from build123d import *

# Parameters (mm, degrees)
SKETCH2_W           = 40
SKETCH2_H           = 25
BOSS_EXTRUDE1_DEPTH = 15
SKETCH3_W           = 25
SKETCH3_H           = 12
CUT_EXTRUDE1_DEPTH  = 5
CUT_EXTRUDE2_DEPTH  = 4.8
SKETCH7_W           = 40
SKETCH7_H           = 25
CUT_EXTRUDE3_DEPTH  = 5


with BuildPart() as part:
    # Sketch2 → Boss-Extrude1 (new body)
    with BuildSketch(Plane.XY):
        with Locations((2.333785617, 1.285617368)):
            Rectangle(SKETCH2_W, SKETCH2_H)
    extrude(amount=BOSS_EXTRUDE1_DEPTH)

    # Sketch3 → Cut-Extrude1 (cut)
    with BuildSketch(Plane.XY.offset(15)):
        with Locations((-0.166214383, 1.285617368)):
            Rectangle(SKETCH3_W, SKETCH3_H)
    extrude(amount=-CUT_EXTRUDE1_DEPTH, mode=Mode.SUBTRACT)

    # Sketch5 → Cut-Extrude2 (cut)
    with BuildSketch(Plane.XY.offset(10)):
        with BuildLine():
            Line((10.563785617, -1.134382632), (10.563785617, 3.705617368))
            Line((10.563785617, 3.705617368), (-6.554265375, 4.705617368))
            ThreePointArc((-6.554265375, 4.705617368), (-11.666214383, 1.285617368), (-6.554265375, -2.134382632))
            Line((-6.554265375, -2.134382632), (10.563785617, -1.134382632))
        make_face()
    extrude(amount=-CUT_EXTRUDE2_DEPTH, mode=Mode.SUBTRACT)

    # Sketch7 → Cut-Extrude3 (cut)
    with BuildSketch(Plane.XY.offset(15)):
        with Locations((2.333785617, 1.285617368)):
            Rectangle(SKETCH7_W, SKETCH7_H)
    extrude(amount=-CUT_EXTRUDE3_DEPTH, mode=Mode.SUBTRACT)


solid = part.part
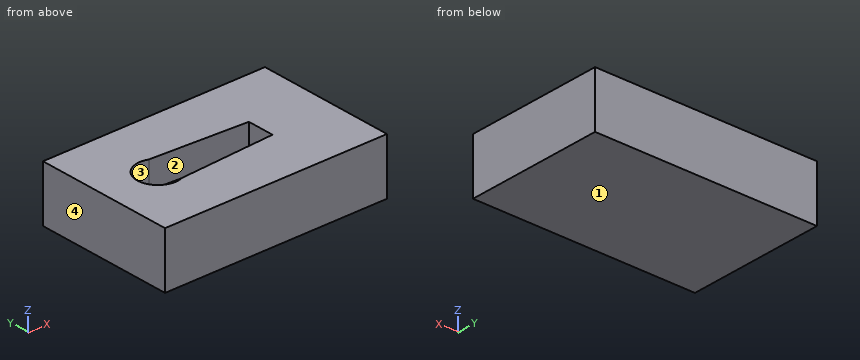
Source: CAD feature listing. Evaluate the final solid. Frame: model axes, mm. Face numbers are marked on the shaded views. Round coordinates to 2 decimals unless told otherwise and drop trailing zeros. Order: outer loops, then holes, each group sorted by start corner. A loop starts at its lowest first (then second) coordinate and runs counter-clockwise, first axis right, second up. Notation, with made-up numbers: (-7, 36) -> (38, 36) arc R13 ccw to (38, 42) -> close; hole circle Ø7 at (-4, 39). An arc over 180 degrees is marked (long way). Answer as CSV lines item,"result".
Item 1: Section A-A, the plane z = 6.75. Return loops of the section in (x, y).
A:
outline,"(-17.67, -11.21) -> (22.33, -11.21) -> (22.33, 13.79) -> (-17.67, 13.79) -> close; hole (-6.55, -2.13) -> (10.56, -1.13) -> (10.56, 3.71) -> (-6.55, 4.71) arc R3.7 ccw (long way) to start"
Item 2: Section C-C, the plane y = 0.5. Return loops of the section in (x, z), plus the area to 3 significant figures.
A:
outline,"(-17.67, 0) -> (22.33, 0) -> (22.33, 10) -> (10.56, 10) -> (10.56, 5.2) -> (-11.58, 5.2) -> (-11.58, 10) -> (-17.67, 10) -> close"
area,"294 mm²"
Item 3: Pull-direction query (X, two-part tool) for the marked faces 1, 2, 3 and 4; classes: pulls with the +X half, pulls with the -X half, needs draft (parallel to the pull), parting line crosses it, or undercut.
A:
face 1,"needs draft"
face 2,"undercut"
face 3,"undercut"
face 4,"pulls with the -X half"
Item 4: Line query: L1, parallel to Z at x = -11, y = 1.75; L2, parallel to X at y = 2.25, z = 9.5; L3, parallel to Y at x = 0, z = 7.25. Output: solid intervals per line, ascending.
A:
L1,"0 to 5.2"
L2,"-17.67 to -11.54, 10.56 to 22.33"
L3,"-11.21 to -1.75, 4.32 to 13.79"
Item 5: Section B-B, the plane x = -8.5. Return loops of the section in (y, z).
A:
outline,"(-11.21, 0) -> (13.79, 0) -> (13.79, 10) -> (4.95, 10) -> (4.95, 5.2) -> (-2.38, 5.2) -> (-2.38, 10) -> (-11.21, 10) -> close"
Item 6: Pin query (flat end, axial travel): pin 1 Ø6 at (x, y) = (-7.97, 1.29) entering from +Z. Return the tip coordinate at first contact, or that it passes through.
A:
pin 1,"z = 5.2"
